Verification items for the finished model (mm, model axes). Round coordinates to 2 decimals unless told otherwise and drop trailing zeros. Loops run counter-clockwise (first coordinate to the right, second up) from the corner with the lowest first, then second, coordinate; pieces in that order, holes last. Notation, with made-up numbers: (25.25, 80) -> (41.25, 80) arc R13 cw to (41.25, 86) -> close; hole circle Ø5 at (8.5, -14). An arc over 180 degrees is marked (long way). Write item = value, one per line.
```python
from build123d import *

# Parameters (mm, degrees)
SKIZZE1_W                       = 200
SKIZZE1_H                       = 200
AUFSATZ_LINEAR_AUSTRAGEN1_DEPTH = 50
VERRUNDUNG1_R                   = 20


with BuildPart() as part:
    # Skizze1 → Aufsatz-Linear austragen1 (new body)
    with BuildSketch(Plane(origin=(0, 0, 0), x_dir=(1, 0, 0), z_dir=(0, 1, 0))):
        Rectangle(SKIZZE1_W, SKIZZE1_H)
    extrude(amount=AUFSATZ_LINEAR_AUSTRAGEN1_DEPTH)

    # Verrundung1
    verrundung1_edges = [part.edges().sort_by_distance(p)[0] for p in [
        (-100, 50, 0),
        (0, 50, 100),
        (100, 50, 0),
        (0, 0, 100),
        (-100, 0, 0),
        (0, 0, -100),
        (100, 0, 0),
        (100, 25, 100),
        (-100, 25, 100),
        (-100, 25, -100),
        (100, 25, -100),
        (0, 50, -100),
    ]]
    fillet(verrundung1_edges, radius=VERRUNDUNG1_R)


solid = part.part
```
(1) Sectioned sample at A-A, the plane x = -65. Record the cut outline in (y, z), and give its area (3 significant figures).
Filled sheet:
outline = (0, -80) arc R20 ccw to (20, -100) -> (30, -100) arc R20 ccw to (50, -80) -> (50, 80) arc R20 ccw to (30, 100) -> (20, 100) arc R20 ccw to (0, 80) -> close
area = 9,660 mm2
(2) Sectioned sample at B-B, the plane z = -86. Record the cut outline in (x, y), and give its area (3 significant figures).
Filled sheet:
outline = (-99.08, 20) arc R19.08 ccw to (-80, 0.92) -> (80, 0.92) arc R19.08 ccw to (99.08, 20) -> (99.08, 30) arc R19.08 ccw to (80, 49.08) -> (-80, 49.08) arc R19.08 ccw to (-99.08, 30) -> close
area = 9,230 mm2
(3) Material ranges on probe 1 along X at (y, z) = (19.5, -78); probe 2 along X at (y, z) = (38, -60); probe 3 along Z at (x, y) = (14.5, 16.5), recorded low to high. Write a range as from..to.
Filled sheet:
probe_1 = -99.99..99.99
probe_2 = -98.33..98.33
probe_3 = -99.69..99.69
(4) Go/stop test with flat-tipped pins: pin 1 Ø4 at (x, y) = (-26.5, 14.5) entering from -Z; pin 2 Ø3 at (y, z) = (16, 45) entering from -X; pin 3 Ø6 at (x, y) = (77.5, 12.5) entering from +Z. Record where each tip stops, or that it passes through.
Filled sheet:
pin_1 = -99.69
pin_2 = -99.84
pin_3 = 99.49
